from build123d import *

# Parameters (mm, degrees)
F0_W     = 9
F0_H     = 38
F0_W_2   = 20
F0_H_2   = 12
F1_DEPTH = 10
F2_DEPTH = 20
F3_DEPTH = 36


with BuildPart() as f1:
    # F0 (on Top) → F1 (new body)
    with BuildSketch(Plane.XY):
        with Locations((4.5, 19)):
            Rectangle(F0_W, F0_H)
        with Locations((40, 44)):
            Rectangle(F0_W_2, F0_H_2)
        Polygon((0, 50), (0, 38), (9, 38), (30, 38), (30, 50), align=None)
        Polygon((9, 38), (9, 0), (30, 0), (30, 20), (50, 20), (50, 38), (30, 38), align=None)
    extrude(amount=F1_DEPTH)

    # F0 (on Top) → F2 (join)
    with BuildSketch(Plane.XY):
        with Locations((4.5, 19)):
            Rectangle(F0_W, F0_H)
        Polygon((0, 50), (0, 38), (9, 38), (30, 38), (30, 50), align=None)
        with Locations((40, 44)):
            Rectangle(F0_W_2, F0_H_2)
    extrude(amount=F2_DEPTH)

    # F0 (on Top) → F3 (join)
    with BuildSketch(Plane.XY):
        Polygon((0, 50), (0, 38), (9, 38), (30, 38), (30, 50), align=None)
    extrude(amount=F3_DEPTH)


solid = f1.part
Part model, mm, in its own coordinate system. A direction names the side the tool comes from. Coordinates: 2 decimals unless noted, no trailing zeros. Write each loop counter-clockwise with the first axis right and the second up, starting at its lowest first coordinate (ties: lowest second). Pieces come first, ordered by that corner, then holes. Notation, with made-up numbers: (-16.75, 60.5) - (32.25, 60.5) arc R10 cw to (32.25, 77.5) - close; hole circle Ø10 at (13.25, -13.75). An arc over 180 degrees is marked (long way). Put each result on its own line as item: value.
1. Band-saw the part on B-B (z = 6.5). Write the cut outline in (x, y).
Final values:
outline: (0, 0) - (30, 0) - (30, 20) - (50, 20) - (50, 50) - (0, 50) - close
2. Band-saw the part on A-A (x = 14). Write the cut outline in (y, z).
Final values:
outline: (0, 0) - (50, 0) - (50, 36) - (38, 36) - (38, 10) - (0, 10) - close
3. Flat gauge pins, fed straight in: pin 1 Ø11 at (x, z) = (36, 6) entering from -Y; pin 2 Ø3.5 at (y, z) = (46.5, 26) entering from +X; pin 3 Ø3.5 at (x, y) = (42.5, 43.5) entering from +Z. Where does each tip first touch, or does it go through?
Final values:
pin 1: stops at y = 20
pin 2: stops at x = 30
pin 3: stops at z = 20
4. Band-saw the part on C-C (z = 24). Write the cut outline in (x, y).
Final values:
outline: (0, 38) - (30, 38) - (30, 50) - (0, 50) - close
5. Probe line 1 along Z through (x, y) = (3.5, 35.5); line 2 along Z through (x, y) = (44.5, 30); line 3 along Y through (x, z) = (37.5, 14.5). List the from-to ranges inside material, lowest first. Write a range as [from, to].
Final values:
line 1: z = [0, 20]
line 2: z = [0, 10]
line 3: y = [38, 50]
6. 3-axis set-ups, long thin cutter, end or side, ignore diameter. For faces 1 (the flat face through (9, 19, 15)), 2 (the flat face through (40, 44, 20)), 3 (the flat face through (50, 38, 8)), 4 (the flat face through (4, 19, 20)), 5 (the flat face through (40, 20, 5)): which of +Z, -Z, +X, -X, +Y, -Y reach the whole face in a straight line?
Final values:
face 1: +Z, +X, -Y
face 2: +Z, +X, +Y, -Y
face 3: +Z, -Z, +X, +Y, -Y
face 4: +Z, +X, -X, -Y
face 5: +Z, -Z, +X, -Y
